from build123d import *

# Parameters (mm, degrees)
EXTRUDE_1_DEPTH     = 350
SKETCH_2_R          = 6
CUT_EXTRUDE_1_DEPTH = 355.541958025
SKETCH_3_R          = 6
CUT_EXTRUDE_2_DEPTH = 355.541958025
SKETCH_4_R          = 6
CUT_EXTRUDE_3_DEPTH = 355.541958025
SKETCH_6_R          = 6
CUT_EXTRUDE_4_DEPTH = 355.541958025


with BuildPart() as part:
    # Эскиз1 → Бобышка-Вытянуть1 (new body)
    with BuildSketch(Plane(origin=(0, 0, 0), x_dir=(0, 0, -1), z_dir=(1, 0, 0))):
        Polygon((0, 0), (0, 40), (4, 40), (4, 4), (40, 4), (40, 0), align=None)
    extrude(amount=EXTRUDE_1_DEPTH)

    # Эскиз2 → Вырез-Вытянуть1 (cut, through all)
    with BuildSketch(Plane.XY):
        with Locations((60, 20)):
            Circle(SKETCH_2_R)
    extrude(amount=-CUT_EXTRUDE_1_DEPTH, mode=Mode.SUBTRACT)

    # Эскиз3 → Вырез-Вытянуть2 (cut, through all)
    with BuildSketch(Plane.XY):
        with Locations((290, 20)):
            Circle(SKETCH_3_R)
    extrude(amount=-CUT_EXTRUDE_2_DEPTH, mode=Mode.SUBTRACT)

    # Эскиз4 → Вырез-Вытянуть3 (cut, through all)
    with BuildSketch(Plane.XY):
        with Locations((240, 20)):
            Circle(SKETCH_4_R)
    extrude(amount=-CUT_EXTRUDE_3_DEPTH, mode=Mode.SUBTRACT)

    # Эскиз6 → Вырез-Вытянуть4 (cut, through all)
    with BuildSketch(Plane.XY):
        with Locations((110, 20)):
            Circle(SKETCH_6_R)
    extrude(amount=-CUT_EXTRUDE_4_DEPTH, mode=Mode.SUBTRACT)


solid = part.part
CAD build for the part. Positions are in the model's coordinates, mm. A direction names the side the tool comes from. Give positions to 0.01 mm unless a question says otherwise; leave off trailing zeros. Write each loop counter-clockwise with the first axis right and the second up, starting at its lowest first coordinate (ties: lowest second). Pieces come first, ordered by that corner, then holes. Notation, with made-up numbers: (77.25, 46.25) -> (117.25, 46.25) arc R17 cw to (117.25, 55.25) -> close; hole circle Ø10 at (-22, -12.5). An arc over 180 degrees is marked (long way). Return JSON: item names as keys, results as strings.
Item 1: Tool access for faces 4 (the cylindrical face through (104, 20, -2)), 5 (the flat face through (173, 4, -22)): list every direction of +Z, -Z, +X, -X, +Y, -Y with a clear straight run to the whole face (end or side of a thin tool).
Answer below:
{"face 4": "+Z, -Z", "face 5": "-Z, +X, -X, +Y"}
Item 2: Two-plate mould, pull along X, no slides. Class faces 1 (the flat face through (350, 3.8, -11.2)), 2 (the cylindrical face through (54, 20, -2)), 3 (the flat face through (173, 22, -4)): +X half, -X half, draft (parallel to the pull), parting line (faces both ways), or undercut.
Answer below:
{"face 1": "+X half", "face 2": "undercut", "face 3": "draft"}
Item 3: Drop flat-ended pins along their axis: pin 1 (14 mm diameter, centred on x = 60, y = 20, fed in from -Z); pin 2 (15.5 mm diameter, centred on x = 110, y = 20, fed in from +Z); pin 3 (7 mm diameter, centred on x = 240, y = 20, fed in from -Z); pin 4 (2 mm diameter, centred on x = 230.5, z = -25, fed in from +Y). Give the stop position or say it passes through.
Answer below:
{"pin 1": "stops at z = -4", "pin 2": "stops at z = 0", "pin 3": "passes through", "pin 4": "stops at y = 4"}
Item 4: Drill centre lines: probe 1 along Y at (x, z) = (60, -2.45); probe 2 along Z at (x, y) = (241.5, 7); probe 3 along Y at (x, z) = (121, -21.5). Where is each one in solid material? Low to high.
Answer below:
{"probe 1": "y = 0 to 14, 26 to 40", "probe 2": "z = -4 to 0", "probe 3": "y = 0 to 4"}
Item 5: Band-saw the part on D-D (z = -26). List the corners of the cut face in (x, y).
Answer below:
{"outline": "(0, 0) -> (350, 0) -> (350, 4) -> (0, 4) -> close"}
Item 6: Band-saw the part on A-A (x = 240). List the corners of the cut face in (y, z).
Answer below:
{"outline": "(0, -40) -> (4, -40) -> (4, -4) -> (14, -4) -> (14, 0) -> (0, 0) -> close; (26, -4) -> (40, -4) -> (40, 0) -> (26, 0) -> close"}
Item 7: Band-saw the part on C-C (x = 80). List the corners of the cut face in (y, z), then the cut area to 3 significant figures.
Answer below:
{"outline": "(0, -40) -> (4, -40) -> (4, -4) -> (40, -4) -> (40, 0) -> (0, 0) -> close", "area": "304 mm2"}
Item 8: Band-saw the part on B-B (y = 20). List the corners of the cut face in (x, z), then the cut area to 3 significant figures.
Answer below:
{"outline": "(0, -4) -> (54, -4) -> (54, 0) -> (0, 0) -> close; (66, -4) -> (104, -4) -> (104, 0) -> (66, 0) -> close; (116, -4) -> (234, -4) -> (234, 0) -> (116, 0) -> close; (246, -4) -> (284, -4) -> (284, 0) -> (246, 0) -> close; (296, -4) -> (350, -4) -> (350, 0) -> (296, 0) -> close", "area": "1,210 mm2"}
